Read the model definition and answer for the solid it produces. Units are mm, in the model's axes. A direction names the side the tool comes from. Coordinates: 2 decimals unless noted, no trailing zeros. Order: outer loops, then holes, each group sorted by start corner. A loop starts at its lowest first (then second) coordinate and runs counter-clockwise, first axis right, second up.
```python
from build123d import *

# Parameters (mm, degrees)
SKETCH_1_R      = 11.25
SKETCH_1_R_2    = 1.5
SKETCH_1_W      = 10
SKETCH_1_H      = 5
EXTRUDE_2_DEPTH = 5


with BuildPart() as part:
    # 草图1 → 凸台-拉伸2 (new body)
    with BuildSketch(Plane(origin=(0, 0, 0), x_dir=(1, 0, 0), z_dir=(0, 1, 0))):
        with BuildLine():
            Line((10, 5), (10, 10))
            Line((10, 10), (30, 10))
            Line((30, 10), (30, 5))
            ThreePointArc((30, 5), (31.464466094, 1.464466094), (35, 0))
            Line((35, 0), (40, 0))
            Line((40, 0), (40, 115))
            Line((40, 115), (45, 115))
            Line((45, 115), (45, 125))
            Line((45, 125), (40, 125))
            Line((40, 125), (40, 135))
            Line((40, 135), (45, 135))
            Line((45, 135), (45, 145))
            Line((45, 145), (40, 145))
            Line((40, 145), (40, 150))
            Line((40, 150), (35, 150))
            Line((35, 150), (35, 145))
            Line((35, 145), (25, 145))
            Line((25, 145), (25, 150))
            Line((25, 150), (20, 150))
            ThreePointArc((20, 150), (5.857864376, 144.142135624), (0, 130))
            Line((0, 130), (0, 0))
            Line((0, 0), (5, 0))
            ThreePointArc((5, 0), (8.535533906, 1.464466094), (10, 5))
        make_face()
        with Locations(Location((20, 106, 0), (0, 0, 270))):
            Circle(SKETCH_1_R, mode=Mode.SUBTRACT)
        with Locations(Location((4.5, 121.5, 0), (0, 0, 270))):
            Circle(SKETCH_1_R_2, mode=Mode.SUBTRACT)
        with Locations(Location((35.5, 121.5, 0), (0, 0, 270))):
            Circle(SKETCH_1_R_2, mode=Mode.SUBTRACT)
        with Locations(Location((4.5, 90.5, 0), (0, 0, 270))):
            Circle(SKETCH_1_R_2, mode=Mode.SUBTRACT)
        with Locations(Location((35.5, 90.5, 0), (0, 0, 270))):
            Circle(SKETCH_1_R_2, mode=Mode.SUBTRACT)
        with Locations((10, 78.5)):
            Rectangle(SKETCH_1_W, SKETCH_1_H, mode=Mode.SUBTRACT)
        with Locations((30, 78.5)):
            Rectangle(SKETCH_1_W, SKETCH_1_H, mode=Mode.SUBTRACT)
    extrude(amount=EXTRUDE_2_DEPTH)


solid = part.part
```
1) Flat-ended cylindrical pins translate along their axes: pin 1 Ø2.5 at (x, y) = (9.5, 1.5) entering from +Z; pin 2 Ø2.5 at (x, y) = (41.5, 2) entering from -Z; pin 3 Ø2.5 at (x, y) = (42, 1.5) entering from +Z; pin 4 Ø4 at (x, z) = (4.5, -90.5) entering from +Y. Find the tip coordinate at first contact, or state that the pin passes through.
A:
pin 1: stops at z = -1.2
pin 2: stops at z = -145
pin 3: stops at z = -115
pin 4: stops at y = 5
2) A cutting plane is placed at B-B, the plane z = -121.5. Determine the outline of the cut face in (x, y), and give its area (3 significant figures).
A:
outline: (0, 0) - (3, 0) - (3, 5) - (0, 5) - close; (6, 0) - (34, 0) - (34, 5) - (6, 5) - close; (37, 0) - (45, 0) - (45, 5) - (37, 5) - close
area: 195 mm2
3) Determine the mould class of faces 5 (the flat face through (43, 2, -125)), 6 (the flat face through (38, 2, -150)), 7 (the flat face through (25, 2, -147)) for opening direction Z: pulls with the +Z half, pulls with the -Z half, needs draft (parallel to the pull), parting line crosses it, or undercut.
A:
face 5: undercut
face 6: pulls with the -Z half
face 7: needs draft
4) A cutting plane is placed at A-A, the plane z = -106. Determine the outline of the cut face in (x, y).
A:
outline: (0, 0) - (8.75, 0) - (8.75, 5) - (0, 5) - close; (31.25, 0) - (40, 0) - (40, 5) - (31.25, 5) - close
5) Which of the six approach directions +Z, -Z, +X, -X, +Y, -Y give full straight-line access (tool end or side, diameter ignored) to faces 1 (the flat face through (40, 2, -57)), 2 (the flat face through (30, 2, -81)), 3 (the flat face through (42, 2, -135)), 4 (the flat face through (30, 2, -8))?
A:
face 1: +Z, +X, +Y, -Y
face 2: +Y, -Y
face 3: +X, +Y, -Y
face 4: +Z, +Y, -Y
6) A cutting plane is placed at C-C, the plane y = 2.55. State how many separate pieces and enclosed holes the cut face has, and give its area (3 significant figures).
A:
separate pieces: 1
enclosed holes: 7
area: 5,230 mm2
7) Straight lines are drawn through the part: line 1 (X direction, y = 1.3, z = -121.5); line 2 (X direction, y = 2.35, z = -90.5); line 3 (Z direction, x = 28.5, y = 1.65). For each, find the intervals that lie inside material, in ascending order.
A:
line 1: x = 0 to 3, 6 to 34, 37 to 45
line 2: x = 0 to 3, 6 to 34, 37 to 40
line 3: z = -145 to -113.37, -98.63 to -81, -76 to -10
8) A cutting plane is placed at D-D, the plane z = -90.5. Determine the outline of the cut face in (x, y).
A:
outline: (0, 0) - (3, 0) - (3, 5) - (0, 5) - close; (6, 0) - (34, 0) - (34, 5) - (6, 5) - close; (37, 0) - (40, 0) - (40, 5) - (37, 5) - close
